```python
from build123d import *

# Parameters (mm, degrees)
SKETCH_W     = 70
SKETCH_H     = 40
SKETCH_R     = 1.5
PAD_DEPTH    = 3
POCKET_DEPTH = 1
FILLET_R     = 3


with BuildPart() as part:
    # Sketch → Pad (new body)
    with BuildSketch(Plane.XY):
        Rectangle(SKETCH_W, SKETCH_H)
        with Locations((-32, 17)):
            Circle(SKETCH_R, mode=Mode.SUBTRACT)
        with Locations((-32, -17)):
            Circle(SKETCH_R, mode=Mode.SUBTRACT)
        with Locations((32, -17)):
            Circle(SKETCH_R, mode=Mode.SUBTRACT)
        with Locations((32, 17)):
            Circle(SKETCH_R, mode=Mode.SUBTRACT)
        Polygon((-32, 11.5), (-32, -11.5), (-26.9, -11.5), (-26.9, -16.5), (26.9, -16.5), (26.9, -11.5), (32, -11.5), (32, 11.5), (26.9, 11.5), (26.9, 16.5), (-26.9, 16.5), (-26.9, 11.5), align=None, mode=Mode.SUBTRACT)
    extrude(amount=PAD_DEPTH)

    # Sketch001 → Pocket (cut)
    with BuildSketch(Plane.XY.offset(3)):
        Polygon((-27.9, 17.8), (27.9, 17.8), (27.9, 12.7), (33, 12.7), (33, -12.7), (27.9, -12.7), (27.9, -17.8), (-27.9, -17.8), (-27.9, -12.7), (-33, -12.7), (-33, 12.7), (-27.9, 12.7), align=None)
    extrude(amount=-POCKET_DEPTH, mode=Mode.SUBTRACT)

    # Fillet
    fillet_edges = [part.edges().sort_by_distance(p)[0] for p in [
        (-35, -20, 1.5),
        (35, -20, 1.5),
        (35, 20, 1.5),
        (-35, 20, 1.5),
    ]]
    fillet(fillet_edges, radius=FILLET_R)


solid = part.part
```
Here's how the part is built. I have some questions about the finished solid (model axes, mm). A direction names the side the tool comes from. Round coordinates to 2 decimals unless told otherwise and drop trailing zeros. Loops run counter-clockwise (first coordinate to the right, second up) from the corner with the lowest first, then second, coordinate; pieces in that order, holes last. Notation, with made-up numbers: (16.25, 60) -> (57.25, 60) arc R18 ccw to (57.25, 93) -> close; hole circle Ø1 at (87, 41.25). An arc over 180 degrees is marked (long way). Answer as CSV lines item,"result". Start each with the question number.
1. For faces 5 (the face through (0, -16.5, 1)), 6 (the face through (35, 0, 1)), which set-ups out of +Z, -Z, +X, -X, +Y, -Y let a thin tool reach every point of the face, with its end or its side?
2. Imagine slicing it at C-C on z = 0.5. Write out the boundary of the cut face in (x, y).
3. Imagine slicing it at A-A on y = -14. Write out the boundary of the cut face in (x, z).
4. I need wall thicknesses on probe 1 along Y at (x, z) = (32, 2.1); probe 2 along Y at (x, z) = (26.5, 0.55); probe 3 along X at (y, z) = (5.5, 0.5). Which ranges of each line are inside material? Lowest first, please. Write a range as from..to.
5. If we mould it in two halves opening along Y, with no side actions, what happens to faces 1 (the face through (-32, 0, 1)), 2 (the face through (-26.9, 14, 1)), 3 (the face through (-5, 18, 3)), 4 (the face through (0, -20, 1))? For each: pulls with the +Y half, pulls with the -Y half, needs draft (parallel to the pull), parting line crosses it, or undercut.
6. Imagine slicing it at B-B on x = 15. Write out the boundary of the cut face in (y, z), plus the area to 3 significant figures.
Solution:
1,face 5,"+Z, -Z"
1,face 6,"+Z, -Z, +X, +Y, -Y"
2,outline,"(-35, -17) arc R3 ccw to (-32, -20) -> (32, -20) arc R3 ccw to (35, -17) -> (35, 17) arc R3 ccw to (32, 20) -> (-32, 20) arc R3 ccw to (-35, 17) -> close; hole circle Ø3 at (-32, -17); hole circle Ø3 at (-32, 17); hole (-32, -11.5) -> (-26.9, -11.5) -> (-26.9, -16.5) -> (26.9, -16.5) -> (26.9, -11.5) -> (32, -11.5) -> (32, 11.5) -> (26.9, 11.5) -> (26.9, 16.5) -> (-26.9, 16.5) -> (-26.9, 11.5) -> (-32, 11.5) -> close; hole circle Ø3 at (32, -17); hole circle Ø3 at (32, 17)"
3,outline,"(-35, 0) -> (-26.9, 0) -> (-26.9, 2) -> (-27.9, 2) -> (-27.9, 3) -> (-35, 3) -> close; (26.9, 0) -> (35, 0) -> (35, 3) -> (27.9, 3) -> (27.9, 2) -> (26.9, 2) -> close"
4,probe 1,"-20..-18.5, -15.5..-12.7, 12.7..15.5, 18.5..20"
4,probe 2,"-20..-16.5, 16.5..20"
4,probe 3,"-35..-32, 32..35"
5,face 1,"undercut"
5,face 2,"undercut"
5,face 3,"needs draft"
5,face 4,"pulls with the -Y half"
6,outline,"(-20, 0) -> (-16.5, 0) -> (-16.5, 2) -> (-17.8, 2) -> (-17.8, 3) -> (-20, 3) -> close; (16.5, 0) -> (20, 0) -> (20, 3) -> (17.8, 3) -> (17.8, 2) -> (16.5, 2) -> close"
6,area,"18.4 mm²"
